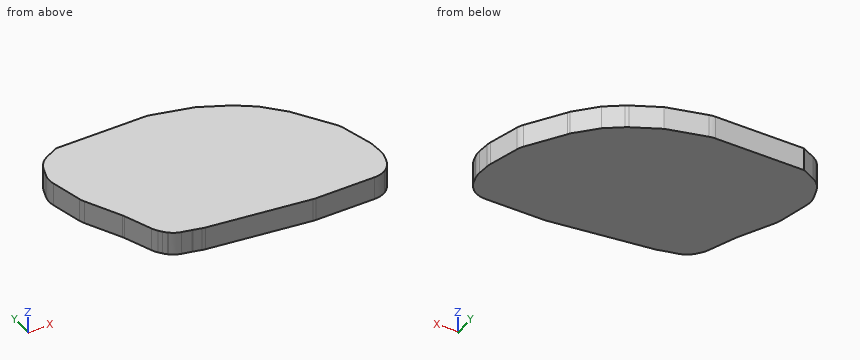
from build123d import *

# Parameters (mm, degrees)
BOSS_EXTRUDE1_DEPTH = 4
SCALE4_SCALE        = 0.75919
FILLET6_R           = 3
FILLET7_R           = 3


with BuildPart() as part:
    # Sketch1 → Boss-Extrude1 (new body)
    with BuildSketch(Plane.XY):
        Polygon((139.887521377, 204.056894723), (141.24778548, 208.242322731), (144.835713473, 210.070135105), (160.500754315, 210.070135105), (167.622266071, 208.242322731), (172.522669487, 205.831679823), (175.619724447, 203.675502319), (178.946764591, 200.233807794), (179.037084843, 200.056512483), (183.5160481, 193.501931379), (185.301557704, 187.487393826), (185.539112291, 184.563645059), (184.954362538, 182.355057305), (184.113784767, 181.109966828), (182.651910383, 180.178021908), (181.232301611, 180.178021908), (171.271612606, 180.178021908), (153.63070922, 182.355057305), (151.966131288, 182.789295026), (149.384829279, 183.363134026), (148.208709289, 184.36807152), (147.189516356, 185.643755739), (145.029311699, 190.88387399), (141.644867129, 197.274737006), align=None)
    extrude(amount=BOSS_EXTRUDE1_DEPTH)


with BuildPart() as part_1:
    # Scale4: scaled about (162.417336375, 194.870616826, 2)
    add(part.part.scale(SCALE4_SCALE).moved(Location((39.111718772, 46.926793238, 0.48162))))

    # Fillet6
    # the kernel refuses this fillet: 3 mm, written as the material it adds along each edge
    with BuildSketch(Plane(origin=(175.034883215, 198.80769695, 0.48162), x_dir=(0.5641904622979087, -0.8256446706980383, 0), z_dir=(0, 0, 1))) as fillet6_piece_1_section:
        with BuildLine():
            CenterArc((FILLET6_R * 0.0642311981219, FILLET6_R), FILLET6_R, 262.649743959, 7.350256041)
            Line((-FILLET6_R * 0.063703385216, FILLET6_R * 0.00821739156901), (0, 0))
            Line((0, 0), (FILLET6_R * 0.0642311981219, 0))
        make_face()
    fillet6_piece_1 = extrude(amount=3.03676, mode=Mode.PRIVATE)
    fillet6_piece_1 = split(fillet6_piece_1, bisect_by=Plane(origin=(175.064317261, 198.840916135, 2), z_dir=(-0.7189811970622167, -0.6950295233088893, 0)), keep=Keep.TOP, mode=Mode.PRIVATE)
    add(fillet6_piece_1)
    with BuildSketch(Plane(origin=(154.482885985, 185.698598128, 0.48162), x_dir=(-0.9761697325769959, 0.21700841734954968, 0), z_dir=(0, 0, 1))) as fillet6_piece_2:
        with BuildLine():
            CenterArc((FILLET6_R * 0.0182188067452, FILLET6_R), FILLET6_R, 267.912509474, 2.087490526)
            Line((-FILLET6_R * 0.0182067162065, FILLET6_R * 0.000663629563253), (0, 0))
            Line((0, 0), (FILLET6_R * 0.0182188067452, 0))
        make_face()
    extrude(amount=3.03676)
    with BuildSketch(Plane(origin=(149.216521921, 191.843921532, 0.48162), x_dir=(-0.4680007470830183, 0.8837280694476876, 0), z_dir=(0, 0, 1))) as fillet6_piece_3:
        with BuildLine():
            CenterArc((FILLET6_R * 0.0480422965927, FILLET6_R), FILLET6_R, 264.498987959, 5.501012041)
            Line((-FILLET6_R * 0.0478210380477, FILLET6_R * 0.00460549475516), (0, 0))
            Line((0, 0), (FILLET6_R * 0.0480422965927, 0))
        make_face()
    extrude(amount=3.03676)
    # the kernel refuses this fillet: 3 mm, written as the material it takes off along each edge
    with BuildSketch(Plane(origin=(170.089204221, 203.192146242, -0.085723646), x_dir=(0.8206934047378623, -0.5713688260832711, 0), z_dir=(0, 0, 1))) as fillet6_2_piece_1:
        with BuildLine():
            CenterArc((FILLET6_R * 0.0756458194575, -FILLET6_R), FILLET6_R, 90, 8.651894609)
            Line((-FILLET6_R * 0.0747850106227, -FILLET6_R * 0.0113794634131), (0, 0))
            Line((0, 0), (FILLET6_R * 0.0756458194575, 0))
        make_face()
    extrude(amount=4.171447292, mode=Mode.SUBTRACT)
    with BuildSketch(Plane(origin=(179.790808366, 189.265347757, -0.299334996), x_dir=(0.08098313210757263, -0.9967154720952452, 0), z_dir=(0, 0, 1))) as fillet6_2_piece_2:
        with BuildLine():
            CenterArc((FILLET6_R * 0.104127332747, -FILLET6_R), FILLET6_R, 90, 11.889267137)
            Line((-FILLET6_R * 0.101893551021, -FILLET6_R * 0.0214524051169), (0, 0))
            Line((0, 0), (FILLET6_R * 0.104127332747, 0))
        make_face()
    extrude(amount=4.598669991, mode=Mode.SUBTRACT)
    with BuildSketch(Plane(origin=(179.527221267, 185.368929193, -0.786529904), x_dir=(-0.5595376521790817, -0.8288049322934323, 0), z_dir=(0, 0, 1))) as fillet6_2_piece_3:
        with BuildLine():
            CenterArc((FILLET6_R * 0.169086653883, -FILLET6_R), FILLET6_R, 90, 19.194353316)
            Line((-FILLET6_R * 0.159686919919, -FILLET6_R * 0.0555912234793), (0, 0))
            Line((0, 0), (FILLET6_R * 0.169086653883, 0))
        make_face()
    extrude(amount=5.573059808, mode=Mode.SUBTRACT)
    with BuildSketch(Plane(origin=(178.435267329, 193.831524522, -0.693636489), x_dir=(0.2845900515763164, -0.9586493115544337, 0), z_dir=(0, 0, 1))) as fillet6_2_piece_4:
        with BuildLine():
            CenterArc((FILLET6_R * 0.156700865162, -FILLET6_R), FILLET6_R, 90, 17.811748872)
            Line((-FILLET6_R * 0.149189673688, -FILLET6_R * 0.0479333120825), (0, 0))
            Line((0, 0), (FILLET6_R * 0.156700865162, 0))
        make_face()
    extrude(amount=5.387272977, mode=Mode.SUBTRACT)
    with BuildSketch(Plane(origin=(178.88906303, 184.423668954, -1.075559702), x_dir=(-0.8432271980573246, -0.5375573387615439, 0), z_dir=(0, 0, 1))) as fillet6_2_piece_5:
        with BuildLine():
            CenterArc((FILLET6_R * 0.207623960269, -FILLET6_R), FILLET6_R, 90, 23.458660046)
            Line((-FILLET6_R * 0.190463329283, -FILLET6_R * 0.0826524595894), (0, 0))
            Line((0, 0), (FILLET6_R * 0.207623960269, 0))
        make_face()
    extrude(amount=6.151119404, mode=Mode.SUBTRACT)
    with BuildSketch(Plane(origin=(169.139414347, 183.71614569, 0.020587263), x_dir=(-0.9924710740045749, 0.12247925238261967, 0), z_dir=(0, 0, 1))) as fillet6_2_piece_6:
        with BuildLine():
            CenterArc((FILLET6_R * 0.0614710316153, -FILLET6_R), FILLET6_R, 90, 7.035208973)
            Line((-FILLET6_R * 0.0610082207674, -FILLET6_R * 0.00752892599542), (0, 0))
            Line((0, 0), (FILLET6_R * 0.0614710316153, 0))
        make_face()
    extrude(amount=3.958825474, mode=Mode.SUBTRACT)
    with BuildSketch(Plane(origin=(155.746616905, 185.368929193, -0.015587097), x_dir=(-0.9676172723968424, 0.2524218971470086, 0), z_dir=(0, 0, 1))) as fillet6_2_piece_7:
        with BuildLine():
            CenterArc((FILLET6_R * 0.0662942795425, -FILLET6_R), FILLET6_R, 90, 7.585665015)
            Line((-FILLET6_R * 0.0657141117056, -FILLET6_R * 0.00875140119136), (0, 0))
            Line((0, 0), (FILLET6_R * 0.0662942795425, 0))
        make_face()
    extrude(amount=4.031174193, mode=Mode.SUBTRACT)
    with BuildSketch(Plane(origin=(150.856527695, 187.865676157, -0.587064111), x_dir=(-0.3811282524443585, 0.9245221766884282, 0), z_dir=(0, 0, 1))) as fillet6_2_piece_8:
        with BuildLine():
            CenterArc((FILLET6_R * 0.14249121477, -FILLET6_R), FILLET6_R, 90, 16.21910898)
            Line((-FILLET6_R * 0.136820147731, -FILLET6_R * 0.0397994153417), (0, 0))
            Line((0, 0), (FILLET6_R * 0.14249121477, 0))
        make_face()
    extrude(amount=5.174128222, mode=Mode.SUBTRACT)
    with BuildSketch(Plane(origin=(151.630288778, 186.897189455, -0.231632642), x_dir=(-0.6241891196597051, 0.7812732831080572, 0), z_dir=(0, 0, 1))) as fillet6_2_piece_9:
        with BuildLine():
            CenterArc((FILLET6_R * 0.0951003522105, -FILLET6_R), FILLET6_R, 90, 10.865021551)
            Line((-FILLET6_R * 0.0933955804828, -FILLET6_R * 0.0179260295894), (0, 0))
            Line((0, 0), (FILLET6_R * 0.0951003522104, 0))
        make_face()
    extrude(amount=4.463265283, mode=Mode.SUBTRACT)
    with BuildSketch(Plane(origin=(152.523187313, 186.134250959, -1.386873198), x_dir=(-0.7602667232190712, 0.6496110448304708, 0), z_dir=(0, 0, 1))) as fillet6_2_piece_10:
        with BuildLine():
            CenterArc((FILLET6_R * 0.249132426376, -FILLET6_R), FILLET6_R, 90, 27.978899274)
            Line((-FILLET6_R * 0.220013935166, -FILLET6_R * 0.116879571377), (0, 0))
            Line((0, 0), (FILLET6_R * 0.249132426376, 0))
        make_face()
    extrude(amount=6.773746396, mode=Mode.SUBTRACT)
    with BuildSketch(Plane(origin=(177.779222616, 183.71614569, -1.705674136), x_dir=(-1, 0, 0), z_dir=(0, 0, 1))) as fillet6_2_piece_11:
        with BuildLine():
            CenterArc((FILLET6_R * 0.291639218067, -FILLET6_R), FILLET6_R, 90, 32.517510615)
            Line((-FILLET6_R * 0.245918120694, -FILLET6_R * 0.156772801943), (0, 0))
            Line((0, 0), (FILLET6_R * 0.291639218067, 0))
        make_face()
    extrude(amount=7.411348271, mode=Mode.SUBTRACT)
    with BuildSketch(Plane(origin=(146.647085448, 196.695800825, -0.397967253), x_dir=(0.4680007470830723, -0.8837280694476589, 0), z_dir=(0, 0, 1))) as fillet6_2_piece_12:
        with BuildLine():
            CenterArc((FILLET6_R * 0.117278300393, FILLET6_R), FILLET6_R, 256.622007888, 13.377992112)
            Line((-FILLET6_R * 0.114095932972, FILLET6_R * 0.027135176844), (0, 0))
            Line((0, 0), (FILLET6_R * 0.117278300394, 0))
        make_face()
    extrude(amount=4.795934506, mode=Mode.SUBTRACT)

    # Fillet7
    fillet7_edges = [part_1.edges().sort_by_distance(p)[0] for p in [
        (145.312926127, 201.844747143, 2),
        (146.345625031, 205.022282232, 2),
        (160.962286441, 206.409939108, 2),
        (179.971157433, 187.04566693, 2),
    ]]
    fillet(fillet7_edges, radius=FILLET7_R)


solid = part_1.part
Input: part model. Units: mm. Frame: model coordinates. Give positions to 0.01 mm unless a question says otherwise; leave off trailing zeros. Write each loop counter-clockwise with the first axis right and the second up, starting at its lowest first coordinate (ties: lowest second). Pieces come first, ordered by that corner, then holes. Notation, with made-up numbers: M -38,-9 L 8,-9 A26 cw 8,11 Z; hole C -3.75,-5.5 d9. An arc over 180 degrees is marked long. Write item = value, one per line. Start each with the question number.
1) Material intervals for line 1 along Y through (x, z) = (162, 2.95); line 2 along Y through (x, z) = (156, 1); line 3 along X through (y, z) = (203, 1.2), sorted ascending. Write a range as [from, to].
2) Cut plane B-B on x = 152.5. Return the cut outline in (y, z), then the cut area to 3 significant figures.
3) Cut plane A-A on y = 198. Return the cut outline in (x, z), then the cut area to 3 significant figures.
Solved:
q1.line_1 = [184.6, 206.14]
q1.line_2 = [185.34, 206.41]
q1.line_3 = [145.69, 170.37]
q2.outline = M 186.25,0.48 L 206.41,0.48 L 206.41,3.52 L 186.25,3.52 Z
q2.area = 61.2 mm2
q3.outline = M 146.31,0.48 L 175.59,0.48 L 175.59,3.52 L 146.31,3.52 Z
q3.area = 88.9 mm2
